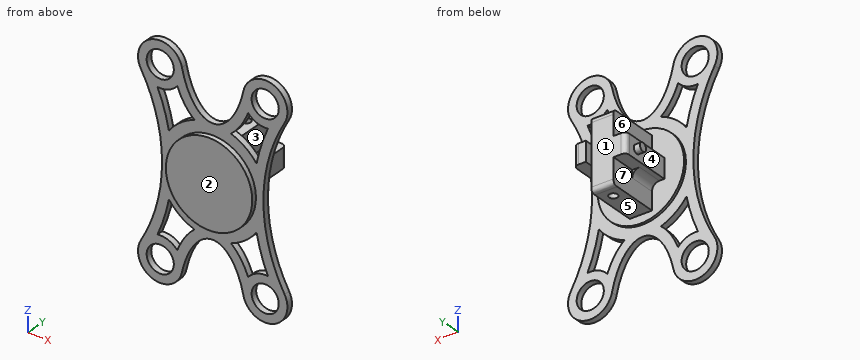
```python
from build123d import *

# Parameters (mm, degrees)
SKETCH1_W                = 100
SKETCH1_H                = 100
BOSS_EXTRUDE1_DEPTH      = 2.5
SKETCH2_W                = 100
SKETCH2_H                = 100
SKETCH2_R                = 5.5
CUT_EXTRUDE1_DEPTH       = 10
CUT_EXTRUDE3_DEPTH       = 10
BOSS_EXTRUDE2_DEPTH      = 1
BOSS_EXTRUDE2_DEPTH_BACK = 4.5
SKETCH6_R                = 17.5
BOSS_EXTRUDE6_DEPTH      = 21
FILLET1_SIZE             = 2
FILLET2_SIZE             = 2
SKETCH12_R               = 1.7
CUT_EXTRUDE4_DEPTH       = 72.5265134
SKETCH13_R               = 1.7
BOSS_EXTRUDE8_DEPTH      = 2.5
SKETCH16_W               = 5
SKETCH16_H               = 8
BOSS_EXTRUDE9_DEPTH      = 24
FILLET3_R                = 2
BOSS_EXTRUDE10_DEPTH     = 10.8


with BuildPart() as part:
    # Sketch1 → Boss-Extrude1 (new body)
    with BuildSketch(Plane(origin=(0, 0, 0), x_dir=(1, 0, 0), z_dir=(0, 1, 0))):
        Rectangle(SKETCH1_W, SKETCH1_H)
    extrude(amount=BOSS_EXTRUDE1_DEPTH)

    # Sketch2 → Cut-Extrude1 (cut)
    # profile 1 of 5: a face of its own
    with BuildSketch(Plane(origin=(0, 2.5, 0), x_dir=(1, 0, 0), z_dir=(0, 1, 0))):
        Rectangle(SKETCH2_W, SKETCH2_H)
        with BuildLine():
            ThreePointArc((-29.074945731, -32.359707621), (-20.523161881, 0), (-29.074945731, 32.359707621))
            ThreePointArc((-29.074945731, 32.359707621), (-24.454355603, 45.216317777), (-12.450207096, 38.693841525))
            add(Edge.make_bspline(
                [(-12.450207096, 38.693841525), (0, -19.342739332), (12.450207096, 38.693841525)],
                knots=[5.128046308, 5.128046308, 5.128046308, 7.438324307, 7.438324307, 7.438324307], degree=2, weights=[1, 0.403791374, 1]))
            ThreePointArc((12.450207096, 38.693841525), (24.454355603, 45.216317777), (29.074945731, 32.359707621))
            ThreePointArc((29.074945731, 32.359707621), (20.523161881, 0), (29.074945731, -32.359707621))
            ThreePointArc((29.074945731, -32.359707621), (24.454355603, -45.216317777), (12.450207096, -38.693841525))
            add(Edge.make_bspline(
                [(12.450207096, -38.693841525), (0, 19.342739332), (-12.450207096, -38.693841525)],
                knots=[5.128046308, 5.128046308, 5.128046308, 7.438324307, 7.438324307, 7.438324307], degree=2, weights=[1, 0.403791374, 1]))
            ThreePointArc((-12.450207096, -38.693841525), (-24.454355603, -45.216317777), (-29.074945731, -32.359707621))
        make_face(mode=Mode.SUBTRACT)
    # profile 2 of 5: a face of its own
    with BuildSketch(Plane(origin=(0, 2.5, 0), x_dir=(1, 0, 0), z_dir=(0, 1, 0))):
        with Locations(Location((-21.25, 36.806079661, 0), (0, 0, 270))):
            Circle(SKETCH2_R)
    # profile 3 of 5: a face of its own
    with BuildSketch(Plane(origin=(0, 2.5, 0), x_dir=(1, 0, 0), z_dir=(0, 1, 0))):
        with Locations(Location((-21.25, -36.806079661, 0), (0, 0, 270))):
            Circle(SKETCH2_R)
    # profile 4 of 5: a face of its own
    with BuildSketch(Plane(origin=(0, 2.5, 0), x_dir=(1, 0, 0), z_dir=(0, 1, 0))):
        with Locations(Location((21.25, -36.806079661, 0), (0, 0, 270))):
            Circle(SKETCH2_R)
    # profile 5 of 5: a face of its own
    with BuildSketch(Plane(origin=(0, 2.5, 0), x_dir=(1, 0, 0), z_dir=(0, 1, 0))):
        with Locations(Location((21.25, 36.806079661, 0), (0, 0, 270))):
            Circle(SKETCH2_R)
    extrude(amount=-CUT_EXTRUDE1_DEPTH, mode=Mode.SUBTRACT)

    # Sketch4 → Cut-Extrude3 (cut)
    with BuildSketch(Plane(origin=(0, 2.5, 0), x_dir=(1, 0, 0), z_dir=(0, 1, 0))):
        with BuildLine():
            ThreePointArc((-17.749489284, -12.998293356), (-13.140045691, -17.64480658), (-7.367625104, -20.729643034))
            add(Edge.make_bspline(
                [(-7.367625104, -20.729643034), (-7.747241798, -21.030061446), (-8.114529726, -21.350348356), (-9.247106431, -22.428016295), (-9.96747496, -23.25295704), (-11.975526868, -25.945450431), (-13.113170007, -28.031524091), (-14.161311212, -30.568863064), (-14.254109179, -30.800153833), (-14.345065296, -31.033569225)],
                knots=[0.658936879, 0.658936879, 0.658936879, 0.658936879, 0.6875, 0.6875, 0.75, 0.75, 0.875, 0.875, 0.887405876, 0.887405876, 0.887405876, 0.887405876], degree=3))
            ThreePointArc((-14.345065296, -31.033569225), (-17.949067849, -28.433275654), (-22.357942029, -27.874536431))
            add(Edge.make_bspline(
                [(-17.749489284, -12.998293356), (-18.730013182, -18.148505445), (-20.279042278, -23.126345909), (-22.357942029, -27.874536431)],
                knots=[0.6784999, 0.6784999, 0.6784999, 0.6784999, 0.896036051, 0.896036051, 0.896036051, 0.896036051], degree=3, weights=[0.94303917, 0.94979881, 0.960677405, 0.975674954]))
        make_face()
        with BuildLine():
            ThreePointArc((7.367625104, -20.729643034), (13.140045691, -17.64480658), (17.749489284, -12.998293356))
            add(Edge.make_bspline(
                [(22.357942029, -27.874536431), (20.279042278, -23.126345909), (18.730013182, -18.148505445), (17.749489284, -12.998293356)],
                knots=[0.103963949, 0.103963949, 0.103963949, 0.103963949, 0.3215001, 0.3215001, 0.3215001, 0.3215001], degree=3, weights=[0.975674954, 0.960677405, 0.94979881, 0.94303917]))
            ThreePointArc((22.357942029, -27.874536431), (17.949067849, -28.433275654), (14.345065296, -31.033569225))
            add(Edge.make_bspline(
                [(14.345065296, -31.033569225), (14.254109179, -30.800153832), (14.161311212, -30.568863064), (13.113170007, -28.031524091), (11.975526868, -25.945450431), (9.96747496, -23.25295704), (9.247106431, -22.428016295), (8.114529726, -21.350348356), (7.747241798, -21.030061447), (7.367625104, -20.729643034)],
                knots=[0.112594124, 0.112594124, 0.112594124, 0.112594124, 0.125, 0.125, 0.25, 0.25, 0.3125, 0.3125, 0.341063121, 0.341063121, 0.341063121, 0.341063121], degree=3))
        make_face()
        with BuildLine():
            ThreePointArc((14.345065296, 31.033569225), (17.949067849, 28.433275654), (22.357942029, 27.874536431))
            add(Edge.make_bspline(
                [(17.749489284, 12.998293356), (18.730013182, 18.148505445), (20.279042278, 23.126345909), (22.357942029, 27.874536431)],
                knots=[0.6784999, 0.6784999, 0.6784999, 0.6784999, 0.896036051, 0.896036051, 0.896036051, 0.896036051], degree=3, weights=[0.94303917, 0.94979881, 0.960677405, 0.975674954]))
            ThreePointArc((17.749489284, 12.998293356), (13.140045691, 17.64480658), (7.367625104, 20.729643034))
            add(Edge.make_bspline(
                [(7.367625104, 20.729643034), (7.747241798, 21.030061446), (8.114529726, 21.350348356), (9.247106431, 22.428016295), (9.96747496, 23.25295704), (11.975526868, 25.945450431), (13.113170007, 28.031524091), (14.161311212, 30.568863064), (14.254109179, 30.800153833), (14.345065296, 31.033569225)],
                knots=[0.658936879, 0.658936879, 0.658936879, 0.658936879, 0.6875, 0.6875, 0.75, 0.75, 0.875, 0.875, 0.887405876, 0.887405876, 0.887405876, 0.887405876], degree=3))
        make_face()
        with BuildLine():
            ThreePointArc((-14.345065296, 31.033569225), (-17.949067849, 28.433275654), (-22.357942029, 27.874536431))
            add(Edge.make_bspline(
                [(-22.357942029, 27.874536431), (-20.279042278, 23.126345909), (-18.730013182, 18.148505445), (-17.749489284, 12.998293356)],
                knots=[0.103963949, 0.103963949, 0.103963949, 0.103963949, 0.3215001, 0.3215001, 0.3215001, 0.3215001], degree=3, weights=[0.975674954, 0.960677405, 0.94979881, 0.94303917]))
            ThreePointArc((-17.749489284, 12.998293356), (-13.140045691, 17.64480658), (-7.367625104, 20.729643034))
            add(Edge.make_bspline(
                [(-14.345065296, 31.033569225), (-14.254109179, 30.800153832), (-14.161311212, 30.568863064), (-13.113170007, 28.031524091), (-11.975526868, 25.945450431), (-9.96747496, 23.25295704), (-9.247106431, 22.428016295), (-8.114529726, 21.350348356), (-7.747241798, 21.030061447), (-7.367625104, 20.729643034)],
                knots=[0.112594124, 0.112594124, 0.112594124, 0.112594124, 0.125, 0.125, 0.25, 0.25, 0.3125, 0.3125, 0.341063121, 0.341063121, 0.341063121, 0.341063121], degree=3))
        make_face()
    extrude(amount=-CUT_EXTRUDE3_DEPTH, mode=Mode.SUBTRACT)

    # Sketch6 → Boss-Extrude2 (add, two sides: drawn at the far end of the back side and taken through both)
    with BuildSketch(Plane(origin=(0, 2.5, 0), x_dir=(1, 0, 0), z_dir=(0, 1, 0)).offset(-BOSS_EXTRUDE2_DEPTH_BACK)):
        with Locations(Location((0, 0, 0), (0, 0, 270))):
            Circle(SKETCH6_R)
    extrude(amount=BOSS_EXTRUDE2_DEPTH + BOSS_EXTRUDE2_DEPTH_BACK)

    # Sketch9 → Boss-Extrude6 (add)
    with BuildSketch(Plane(origin=(0, 3.5, 0), x_dir=(1, 0, 0), z_dir=(0, 1, 0))):
        Polygon((-4.5, 4), (-9.5, 4), (-9.5, -4), (-4.5, -4), (-4.5, -14.2), (4.5, -14.2), (4.5, 14.2), (-4.5, 14.2), align=None)
    extrude(amount=BOSS_EXTRUDE6_DEPTH)

    # Fillet1
    # a fillet whose section is not a circle: 2 mm, written as the material it takes off along each edge
    with BuildSketch(Plane(origin=(-9.5, 24.5, -9), x_dir=(0, -1, 0), z_dir=(0, 0, 1))) as fillet1_piece_1:
        with BuildLine():
            add(Edge.make_bspline([(FILLET1_SIZE, 0), (FILLET1_SIZE * 0.831801948466, 0), (FILLET1_SIZE * 0.663603896932, 0), (FILLET1_SIZE * 0.292893218813, FILLET1_SIZE * 0.0716919198361), (FILLET1_SIZE * 0.0716919198361, FILLET1_SIZE * 0.292893218813), (0, FILLET1_SIZE * 0.663603896932), (0, FILLET1_SIZE * 0.831801948466), (0, FILLET1_SIZE)], knots=[0, 0, 0, 0, 0, 0, 0.5, 0.5, 1, 1, 1, 1, 1, 1], degree=5))
            Line((0, FILLET1_SIZE), (0, 0))
            Line((0, 0), (FILLET1_SIZE, 0))
        make_face()
    extrude(amount=18, mode=Mode.SUBTRACT)

    # Fillet2
    # a fillet whose section is not a circle: 2 mm, written as the material it takes off along each edge
    with BuildSketch(Plane(origin=(-9.5, 24.5, 14.2), x_dir=(0, -1, 0), z_dir=(1, 0, 0)), Plane(origin=(9.5, 24.5, -14.2), x_dir=(0, -1, 0), z_dir=(-1, 0, 0))) as fillet2_piece_1:
        with BuildLine():
            add(Edge.make_bspline([(FILLET2_SIZE, 0), (FILLET2_SIZE * 0.831801948466, 0), (FILLET2_SIZE * 0.663603896932, 0), (FILLET2_SIZE * 0.292893218813, FILLET2_SIZE * 0.0716919198361), (FILLET2_SIZE * 0.0716919198361, FILLET2_SIZE * 0.292893218813), (0, FILLET2_SIZE * 0.663603896932), (0, FILLET2_SIZE * 0.831801948466), (0, FILLET2_SIZE)], knots=[0, 0, 0, 0, 0, 0, 0.5, 0.5, 1, 1, 1, 1, 1, 1], degree=5))
            Line((0, FILLET2_SIZE), (0, 0))
            Line((0, 0), (FILLET2_SIZE, 0))
        make_face()
    extrude(amount=19, mode=Mode.SUBTRACT)

    # Sketch12 → Cut-Extrude4 (cut, through all)
    with BuildSketch(Plane(origin=(0, 0, -14.2), x_dir=(-1, 0, 0), z_dir=(0, 0, -1))):
        with Locations((0, 18.5)):
            Circle(SKETCH12_R)
    extrude(amount=-CUT_EXTRUDE4_DEPTH, mode=Mode.SUBTRACT)

    # Sketch13 → Boss-Extrude8 (add)
    with BuildSketch(Plane.ZY.offset(9.5)):
        with Locations(Location((0, 18.5, 0), (0, 0, 180))):
            Circle(SKETCH13_R)
    extrude(amount=BOSS_EXTRUDE8_DEPTH)

    # Sketch16 → Boss-Extrude9 (add)
    with BuildSketch(Plane(origin=(0, 3.5, 0), x_dir=(1, 0, 0), z_dir=(0, 1, 0))):
        with Locations((7, 0)):
            Rectangle(SKETCH16_W, SKETCH16_H)
    extrude(amount=BOSS_EXTRUDE9_DEPTH)

    # Fillet3
    fillet3_edges = [part.edges().sort_by_distance(p)[0] for p in [
        (9.5, 27.5, 0),
    ]]
    fillet(fillet3_edges, radius=FILLET3_R)

    # Sketch18 → Boss-Extrude10 (add)
    with BuildSketch(Plane(origin=(0, 3.5, 0), x_dir=(1, 0, 0), z_dir=(0, 1, 0))):
        with BuildLine():
            Line((-9.5, -4), (-7.5, -4))
            ThreePointArc((-7.5, -4), (-5.378679656, -4.878679656), (-4.5, -7))
            Line((-4.5, -7), (-4.5, -14.2))
            Line((-4.5, -14.2), (4.5, -14.2))
            Line((4.5, -14.2), (4.5, -7))
            ThreePointArc((4.5, -7), (5.378679656, -4.878679656), (7.5, -4))
            Line((7.5, -4), (9.5, -4))
            Line((9.5, -4), (9.5, 4))
            Line((9.5, 4), (7.5, 4))
            ThreePointArc((7.5, 4), (5.378679656, 4.878679656), (4.5, 7))
            Line((4.5, 7), (4.5, 14.2))
            Line((4.5, 14.2), (-4.5, 14.2))
            Line((-4.5, 14.2), (-4.5, 7))
            ThreePointArc((-4.5, 7), (-5.378679656, 4.878679656), (-7.5, 4))
            Line((-7.5, 4), (-9.5, 4))
            Line((-9.5, 4), (-9.5, -4))
        make_face()
    extrude(amount=BOSS_EXTRUDE10_DEPTH)


solid = part.part
```
The model under review builds one solid part; all positions refer to its coordinate system, in mm. Face numbers are marked on the shaded views. A direction names the side the tool comes from. Round coordinates to 2 decimals unless told otherwise and drop trailing zeros. Loops run counter-clockwise (first coordinate to the right, second up) from the corner with the lowest first, then second, coordinate; pieces in that order, holes last.
Item 1: For line 1 (Y direction, x = 0, z = -0.75); line 2 (Y direction, x = 11.5, z = -34); line 3 (Z direction, x = 1, y = 12), list the stretches that pass through material, from the lowest coordinate up.
Determined:
line 1: y = -2 to 16.8, 20.2 to 24.5
line 2: y = 0 to 2.5
line 3: z = -14.2 to 14.2
Item 2: Mouldability with a two-part tool opening along Y and no side actions: class the marked faces 1, 2, 3 and 4 as released by +Y, released by -Y, zero draft, split by the parting line, or undercut.
Determined:
face 1: released by +Y
face 2: released by -Y
face 3: zero draft
face 4: undercut
Item 3: Take a section at B-B (y = 5.75). Write out the cut boundary in (x, z), then the cut area to 3 significant figures.
Determined:
outline: (-9.5, -4) - (-7.5, -4) arc R3 cw to (-4.5, -7) - (-4.5, -14.2) - (4.5, -14.2) - (4.5, -7) arc R3 cw to (7.5, -4) - (9.5, -4) - (9.5, 4) - (7.5, 4) arc R3 cw to (4.5, 7) - (4.5, 14.2) - (-4.5, 14.2) - (-4.5, 7) arc R3 cw to (-7.5, 4) - (-9.5, 4) - close
area: 343 mm2
Item 4: Take a section at C-C (z = -35). Give the number of separate pieces and of enclosed holes in the cut face, then the cut area to 3 significant figures.
Determined:
separate pieces: 4
enclosed holes: 0
area: 40.9 mm2
Item 5: Take a section at A-A (y = 18.5). Write out the cut boundary in (x, z), then the cut area to 3 significant figures.
Determined:
outline: (-12, -1.7) - (-9.5, -1.7) - (-9.5, -4) - (-4.5, -4) - (-4.5, -14.2) - (-1.7, -14.2) - (-1.7, 14.2) - (-4.5, 14.2) - (-4.5, 4) - (-9.5, 4) - (-9.5, 1.7) - (-12, 1.7) - close; (1.7, -14.2) - (4.5, -14.2) - (4.5, -4) - (9.5, -4) - (9.5, 4) - (4.5, 4) - (4.5, 14.2) - (1.7, 14.2) - close
area: 248 mm2
Item 6: For the marked faces 5, 6 and 7, list the 3-axis set-ups (+Z, -Z, +X, -X, +Y, -Y) from which the entire face can be reached by the end or side of a thin tool; tool diameter is ignored.
Determined:
face 5: -Z, +X, -X, +Y
face 6: +Z, -X, +Y
face 7: -Z, -X, +Y
Item 7: Clearance check with flat-ended pins moving along their axes: pin 1 Ø0.9 at (x, z) = (-6, -6) entering from +Y; pin 2 Ø6 at (x, z) = (-4, -3) entering from +Y; pin 3 Ø11 at (y, z) = (15, 8) entering from -X; pin 4 Ø12 at (x, z) = (22, -6) entering from -Y. State where each tip first meets the part, or that it passes through.
Determined:
pin 1: stops at y = 3.5
pin 2: stops at y = 24.5
pin 3: stops at x = -9.5
pin 4: stops at y = -2
